Geometry: final body of the model. Coordinates: model frame, mm. Give positions to 0.01 mm unless a question says otherwise; leave off trailing zeros. Loops run counter-clockwise (first coordinate to the right, second up) from the corner with the lowest first, then second, coordinate; pieces in that order, holes last. Notation, with made-up numbers: (38, 27) -> (96, 27) arc R14 cw to (96, 33) -> close; hole circle Ø8 at (25, -22.5). An arc over 180 degrees is marked (long way). Answer in a Markdown table with one row per item. Add a question column.
1) Line query: line 1 (Y direction, x = 139, z = 0); line 2 (X direction, y = -29, z = -17.5); line 3 (Y direction, x = 57, z = 5.5). Output: solid intervals per line, ascending. Write a range as from..to.
2) Draft query along Z for faces 1 (the flat face through (189.133, 21, -18)), 2 (the conical face through (13.946, 16.132, 3.582)), 3 (the cylindrical face through (107.92, -27.153, 3.565)), 4 (the conical face through (8.41, -6.7, -21.27)). Return one class per face: +Z half, -Z half, draft (parallel to the pull), parting line (faces both ways), or undercut.
3) Section query A-A (x = 161). Return the cut outline in (y, z), plus the area to 3 significant figures.
4) First-contact query: P1, Ø10, axis at x = 102, z = -4.5, coming from the -Y side; P2, Ø3, axis at x = -1, z = 23, coming from the +Y side; P3, Ø6, axis at y = -20, z = -6.5, coming from the +X side; P4, Ø12, axis at x = 66.5, y = -14, coming from the +Z side. Flat tips, straight axial feed; report the tip coordinate or a pass-through.
```python
from build123d import *


with BuildPart() as part:
    # Sketch1 → Revolve1 (revolve)
    with BuildSketch(Plane.XY, mode=Mode.PRIVATE) as revolve1_sk:
        with BuildLine():
            Line((189.133015331, 27.386004017), (28.949236933, 27.386004017))
            ThreePointArc((28.949236933, 27.386004017), (25.12240261, 26.624799342), (21.878169121, 24.457071829))
            Line((21.878169121, 24.457071829), (13.541703369, 16.120606076))
            ThreePointArc((13.541703369, 16.120606076), (8.091391109, 12.478823854), (1.662309445, 11.2))
            ThreePointArc((1.662309445, 11.2), (0.81433228, 11.284876268), (0, 11.536137468))
            add(Edge.make_bspline(
                [(0, 11.536137468), (-19.948257354, 19.947595697), (-40.127010283, 24.64)],
                knots=[0, 0, 0, 1, 1, 1], degree=2))
            Line((-40.127010283, 24.64), (-38.315022829, 32.432092239))
            add(Edge.make_bspline(
                [(2.348184674, 19.226769399), (-17.827706836, 27.665327765), (-38.315022829, 32.432092239)],
                knots=[0.018493807, 0.018493807, 0.018493807, 1, 1, 1], degree=2))
            ThreePointArc((2.348184674, 19.226769399), (5.344435892, 20.007381854), (7.884849119, 21.777460326))
            Line((7.884849119, 21.777460326), (16.221314872, 30.113926078))
            ThreePointArc((16.221314872, 30.113926078), (22.060935151, 34.015835602), (28.949236933, 35.386004017))
            Line((28.949236933, 35.386004017), (189.133015331, 35.386004017))
            Line((189.133015331, 35.386004017), (189.133015331, 27.386004017))
        make_face()
    revolve(revolve1_sk.sketch.rotate(Axis((0, 0, 0), (-1, 0, 0)), 90), axis=Axis((0, 0, 0), (-1, 0, 0)))


solid = part.part
```
Evaluation:
| question | item | result |
|---|---|---|
| 1 | line 1 | -35.39..-27.39, 27.39..35.39 |
| 1 | line 2 | 21.72..189.13 |
| 1 | line 3 | -34.96..-26.83, 26.83..34.96 |
| 2 | face 1 | draft |
| 2 | face 2 | undercut |
| 2 | face 3 | undercut |
| 2 | face 4 | parting line |
| 3 | outline | circle Ø70.77 at (0, 0); hole circle Ø54.77 at (0, 0) |
| 3 | area | 1,580 mm² |
| 4 | P1 | y = -35.39 |
| 4 | P2 | through |
| 4 | P3 | x = 21.45 |
| 4 | P4 | z = 34.47 |
